```python
from build123d import *

# Parameters (mm, degrees)
CROQUIS1_R              = 21
SALIENTE_EXTRUIR1_DEPTH = 21.4
CROQUIS2_R              = 1.750000001
CROQUIS2_R_2            = 1.75
SALIENTE_EXTRUIR2_DEPTH = 0.8
CROQUIS3_R              = 5
SALIENTE_EXTRUIR3_DEPTH = 1.5
CROQUIS4_R              = 1.5
SALIENTE_EXTRUIR4_DEPTH = 8.5
CROQUIS5_R              = 5
CROQUIS5_R_2            = 1.5
SALIENTE_EXTRUIR5_DEPTH = 5.5
SALIENTE_EXTRUIR6_START = 1
CROQUIS6_R              = 1.5
SALIENTE_EXTRUIR6_DEPTH = 1


with BuildPart() as part:
    # Croquis1 → Saliente-Extruir1 (new body)
    with BuildSketch(Plane(origin=(0, 0, 0), x_dir=(1, 0, 0), z_dir=(0, 1, 0))):
        with Locations(Location((0, 0, 0), (0, 0, 270))):
            Circle(CROQUIS1_R)
    extrude(amount=SALIENTE_EXTRUIR1_DEPTH)

    # Croquis2 → Saliente-Extruir2 (add)
    with BuildSketch(Plane(origin=(0, 21.4, 0), x_dir=(1, 0, 0), z_dir=(0, 1, 0))):
        with BuildLine():
            Line((-27.36337, -2.691836219), (-14.634872681, -15.060561132))
            ThreePointArc((-14.634872681, -15.060561132), (0.00030013, -20.999999998), (14.635303163, -15.060142806))
            Line((14.635303163, -15.060142806), (27.363446993, -2.691054009))
            ThreePointArc((27.363446993, -2.691054009), (27.421544543, 2.629863133), (22.100355918, 2.651912466))
            Line((22.100355918, 2.651912466), (20.946382723, 1.499683579))
            ThreePointArc((20.946382723, 1.499683579), (1e-09, 21), (-20.946382722, 1.499683581))
            Line((-20.946382722, 1.499683581), (-22.101170465, 2.652018145))
            ThreePointArc((-22.101170465, 2.652018145), (-27.421985882, 2.628707389), (-27.36337, -2.691836219))
        make_face()
        with Locations(Location((24.75, -0.001742794, 0), (0, 0, 270))):
            Circle(CROQUIS2_R, mode=Mode.SUBTRACT)
        with Locations(Location((-24.749999879, -0.002450302, 0), (0, 0, 270))):
            Circle(CROQUIS2_R_2, mode=Mode.SUBTRACT)
    extrude(amount=SALIENTE_EXTRUIR2_DEPTH)

    # Croquis3 → Saliente-Extruir3 (add)
    with BuildSketch(Plane(origin=(0, 22.2, 0), x_dir=(1, 0, 0), z_dir=(0, 1, 0))):
        with Locations(Location((0, 0, 0), (0, 0, 270))):
            Circle(CROQUIS3_R)
    extrude(amount=SALIENTE_EXTRUIR3_DEPTH)

    # Croquis4 → Saliente-Extruir4 (add)
    with BuildSketch(Plane(origin=(0, 23.7, 0), x_dir=(1, 0, 0), z_dir=(0, 1, 0))):
        with Locations(Location((0, 0, 0), (0, 0, 270))):
            Circle(CROQUIS4_R)
    extrude(amount=SALIENTE_EXTRUIR4_DEPTH)

    # Croquis5 → Saliente-Extruir5 (add)
    with BuildSketch(Plane(origin=(0, 25.7, 0), x_dir=(1, 0, 0), z_dir=(0, 1, 0))):
        with Locations(Location((0, 0, 0), (0, 0, 270))):
            Circle(CROQUIS5_R)
        with Locations(Location((0, 0, 0), (0, 0, 270))):
            Circle(CROQUIS5_R_2, mode=Mode.SUBTRACT)
    extrude(amount=SALIENTE_EXTRUIR5_DEPTH)

    # Croquis6 → Saliente-Extruir6 (add)
    with BuildSketch(Plane.XZ.offset(SALIENTE_EXTRUIR6_START)):
        with Locations(Location((0, 0, 0), (0, 0, 90))):
            Circle(CROQUIS6_R)
    extrude(amount=-SALIENTE_EXTRUIR6_DEPTH)


solid = part.part
```
Here's how the part is built. I have some questions about the finished solid (model axes, mm). A direction names the side the tool comes from. Round coordinates to 2 decimals unless told otherwise and drop trailing zeros. Order: outer loops, then holes, each group sorted by start corner. A loop starts at its lowest first (then second) coordinate and runs counter-clockwise, first axis right, second up. Notation, with made-up numbers: (-31, 17.25) -> (16, 17.25) arc R9 ccw to (16, 28.25) -> close; hole circle Ø4 at (-31.5, 74). An arc over 180 degrees is marked (long way). Use a Markdown table: item, result. Add a question column.
(1) Suppose I cut it at D-D, the plane z = 10. Please give me the cut outline in (x, y).
(2) For pin 1 Ø2 at (x, z) = (-24.75, 0) entering from +Y; pin 2 Ø1.5 at (x, z) = (11.5, -2) entering from -Y; pin 3 Ø12 at (x, z) = (21.5, 0.5) entering from +Y; pin 4 Ø4.5 at (x, z) = (24.75, 0) entering from -Y, each with a flat end and sliding along its axis, tell me the tip position at first contact or that it passes through.
(3) For faces 5 (the face through (0.45, 24.69, 1.43)), 6 (the face through (1.2, 31.2, -1.2)), 7 (the face through (-26.458, 21.794, -0.377)), 8 (the face through (-21.09, 21.79, 8.79)), 9 (the face through (-0.45, -0.51, 1.43)), which set-ups out of +Z, -Z, +X, -X, +Y, -Y let a thin tool reach every point of the face, with its end or its side?
(4) Suppose I cut it at B-B, the plane x = -24.75. Please give me the cut outline in (y, z).
(5) Suppose I cut it at A-A, the plane x = 0. Please give me the cut outline in (y, z).
(6) I need wall thicknesses on line 1 along Y through (x, z) = (3.5, 1); line 2 along Y through (x, z) = (-6.5, 16.5); line 3 along Z through (x, y) = (24, 22). Which ranges of each line are inside material? Lowest first, please.
(7) Suppose I cut it at C-C, the plane z = 0. Count the separate pieces of the cut face and the enclosed holes in it, and give its area (3 significant figures).
(8) If we mould it in two halves opening along Y, with no side actions, what happens to faces 1 (the face through (6, 22.2, 0)), 2 (the face through (1.2, 23.7, -1.2)), 3 (the face through (1.2, 25.7, -1.2)), 4 (the face through (-4.88, 22.94, -1.08))? For each: released by +Y, released by -Y, zero draft, split by the parting line, or undercut.
Verdict:
| question | item | result |
|---|---|---|
| 1 | outline | (-19.84, 21.4) -> (-18.47, 21.4) -> (-18.47, 0) -> (18.47, 0) -> (18.47, 21.4) -> (19.84, 21.4) -> (19.84, 22.2) -> (-19.84, 22.2) -> close |
| 2 | pin 1 | through |
| 2 | pin 2 | y = 0 |
| 2 | pin 3 | y = 22.2 |
| 2 | pin 4 | y = 21.4 |
| 3 | face 5 | none |
| 3 | face 6 | +Y |
| 3 | face 7 | +Y, -Y |
| 3 | face 8 | +Z, -X, +Y, -Y |
| 3 | face 9 | -Y |
| 4 | outline | (21.4, -3.75) -> (22.2, -3.75) -> (22.2, -1.75) -> (21.4, -1.75) -> close; (21.4, 1.75) -> (22.2, 1.75) -> (22.2, 5.23) -> (21.4, 5.23) -> close |
| 5 | outline | (-1, -1.5) -> (0, -1.5) -> (0, -21) -> (22.2, -21) -> (22.2, -5) -> (23.7, -5) -> (23.7, -1.5) -> (25.7, -1.5) -> (25.7, -5) -> (31.2, -5) -> (31.2, -1.5) -> (32.2, -1.5) -> (32.2, 1.5) -> (31.2, 1.5) -> (31.2, 5) -> (25.7, 5) -> (25.7, 1.5) -> (23.7, 1.5) -> (23.7, 5) -> (22.2, 5) -> (22.2, 21) -> (0, 21) -> (0, 1.5) -> (-1, 1.5) -> close |
| 6 | line 1 | 0 to 23.7, 25.7 to 31.2 |
| 6 | line 2 | 0 to 22.2 |
| 6 | line 3 | -3.67 to -1.58, 1.58 to 5.96 |
| 7 | separate pieces | 3 |
| 7 | enclosed holes | 0 |
| 7 | area | 1,020 mm2 |
| 8 | face 1 | released by +Y |
| 8 | face 2 | undercut |
| 8 | face 3 | undercut |
| 8 | face 4 | zero draft |
